```python
from build123d import *

# Parameters (mm, degrees)
F1_DEPTH = 20


with BuildPart() as f1:
    # F0 (on Front) → F1 (new body)
    with BuildSketch(Plane.XZ):
        Polygon((725.387353, 96.851042), (-734.612647, 96.851042), (-734.612647, 56.851042), (-734.612647, -143.148958), (-724.612647, -143.148958), (-724.612647, 56.851042), (-258.012647, 56.851042), (-258.012647, -143.148958), (-238.012647, -143.148958), (-238.012647, 56.851042), (228.587353, 56.851042), (228.587353, -143.148958), (248.587353, -143.148958), (248.587353, 56.851042), (715.387353, 56.851042), (715.387353, -143.148958), (725.387353, -143.148958), (725.387353, 56.851042), align=None)
        Polygon((-724.612647, -143.148958), (-734.612647, -143.148958), (-734.612647, -163.148958), (725.567341, -163.148958), (725.387353, -143.148958), (715.387353, -143.148958), (248.587353, -143.148958), (228.587353, -143.148958), (-238.012647, -143.148958), (-258.012647, -143.148958), align=None)
    extrude(amount=F1_DEPTH)


solid = f1.part
```
Geometry: final body of the model. Coordinates: model frame, mm. Coordinates: 2 decimals unless noted, no trailing zeros. Order: outer loops, then holes, each group sorted by start corner. A loop starts at its lowest first (then second) coordinate and runs counter-clockwise, first axis right, second up. Notation, with made-up numbers: M 32,86 L 69,86 A9 ccw 69,96 Z; hole C -30.5,7.25 d10. An arc over 180 degrees is marked long. Answer in a Markdown table with one row per item. Add a question column.
Q1. Line query: L1, parallel to X at y = -16.5, z = -110.5; L2, parallel to Z at x = 262, y = -9; L3, parallel to X at y = -7.75, z = 75.5. Output: solid intervals per line, ascending.
Q2. Section query A-A on z = -52. Return the cut outline in (x, y).
Q3. Section query C-C on y = -14.25. Return the cut outline in (x, z), and give its area (3 significant figures).
Q4. Section query B-B on x = -586. Return the cut outline in (y, z), and give its area (3 significant figures).
Q5. Mould query, pull axis Y, two halves, no side actions, for faces 1 (the flat face through (-8, 0, 73)), 2 (the flat face through (-8, -20, 73)). Classes: released by +Y, released by -Y, zero draft, split by the parting line, or undercut.
Completed:
| question | item | result |
|---|---|---|
| 1 | L1 | x = -734.61 to -724.61, -258.01 to -238.01, 228.59 to 248.59, 715.39 to 725.39 |
| 1 | L2 | z = -163.15 to -143.15, 56.85 to 96.85 |
| 1 | L3 | x = -734.61 to 725.39 |
| 2 | outline | M -734.61,-20 L -724.61,-20 L -724.61,0 L -734.61,0 Z; M -258.01,-20 L -238.01,-20 L -238.01,0 L -258.01,0 Z; M 228.59,-20 L 248.59,-20 L 248.59,0 L 228.59,0 Z; M 715.39,-20 L 725.39,-20 L 725.39,0 L 715.39,0 Z |
| 3 | outline | M -734.61,-163.15 L 725.57,-163.15 L 725.39,-143.15 L 725.39,96.85 L -734.61,96.85 Z; hole M -724.61,-143.15 L -258.01,-143.15 L -258.01,56.85 L -724.61,56.85 Z; hole M -238.01,-143.15 L 228.59,-143.15 L 228.59,56.85 L -238.01,56.85 Z; hole M 248.59,-143.15 L 715.39,-143.15 L 715.39,56.85 L 248.59,56.85 Z |
| 3 | area | 99,600 mm2 |
| 4 | outline | M -20,-163.15 L 0,-163.15 L 0,-143.15 L -20,-143.15 Z; M -20,56.85 L 0,56.85 L 0,96.85 L -20,96.85 Z |
| 4 | area | 1,200 mm2 |
| 5 | face 1 | released by +Y |
| 5 | face 2 | released by -Y |
